Autodesk Inventor part; units mm, degrees
ref_plane "YZ Plane" through (0, 0, 0) normal (1, 0, 0) x (0, 1, 0)
ref_plane "XZ Plane" through (0, 0, 0) normal (0, 1, 0) x (-1, 0, 0)
ref_plane "XY Plane" through (0, 0, 0) normal (0, 0, 1) x (1, 0, 0)
sketch "Sketch3" plane through (0, 0, 0) normal (0, 1, 0) x (-1, 0, 0)
  line L0 (-44, 50) -> (44, 50)
  line L1 (44, 50) -> (44, -50)
  line L2 (44, -50) -> (-44, -50)
  line L3 (-44, -50) -> (-44, 50)
  line L4 (-44, 50) -> (44, -50) construction
  line L5 (44, 50) -> (-44, -50) construction
  line L6 (44, 50) -> (-44, 50)
  line L7 (-44, 50) -> (-44, 47)
  line L8 (-44, 47) -> (44, 47)
  line L9 (44, 47) -> (44, 50)
  line L10 (44, 47) -> (41, 47)
  line L11 (41, 47) -> (41, -50)
  line L12 (41, -50) -> (44, -50)
  line L13 (44, -50) -> (44, 47)
  line L14 (-44, 47) -> (-41, 47)
  line L15 (-41, 47) -> (-41, -50)
  line L16 (-41, -50) -> (-44, -50)
  line L17 (-44, -50) -> (-44, 47)
  line L18 (41, -50) -> (-41, -50)
  line L19 (-41, -50) -> (-41, -47)
  line L20 (-41, -47) -> (41, -47)
  line L21 (41, -47) -> (41, -50)
  line L22 (41, 47) -> (34, 47)
  line L23 (34, 47) -> (34, -50)
  line L24 (34, -50) -> (37, -50)
  line L25 (37, -50) -> (37, 50)
  line L26 (34, 47) -> (34, 50)
  line L27 (41, 47) -> (41, 50)
  line L28 (-41, 47) -> (-41, 50)
  point P0 (0, 0)
  point P1 (37, -47)
  point P2 (37, 47)
  point P3 (34, -47)
  point P4 (37, 50)
  dimension "d33" = 88
  dimension "d34" = 100
  dimension "d35" = 88
  dimension "d36" = 3
  dimension "d37" = 3
  dimension "d38" = 3
  dimension "d39" = 3
  dimension "d63" = 7
  dimension "d64" = 3
extrude "Extrusion2" add sketch "Sketch3" along normal blind 100 contours L8 L15 L2 L3 | L8 L25 L20 L23 | L20 L23 L2 L15 | L20 L25 L2 L23
sketch "Sketch6" plane through (44, 0, -50) normal (0, 0, -1) x (-1, 0, 0)
  circle A0 centre (62.07, 7.54) radius 1.5875
  circle A1 centre (10, 12.62) radius 1.5875
  circle A2 centre (10, 40.56) radius 1.5875
  line L0 (7.46, 10.08) -> (7.46, 42.846)
  line L1 (7.46, 42.846) -> (10, 45.386)
  line L2 (10, 45.386) -> (10, 58.34)
  line L3 (10, 7.54) -> (7.46, 10.08)
  line L4 (10, 5) -> (10, 7.54)
  line L5 (76.04, 5) -> (10, 5)
  line L6 (76.04, 58.34) -> (76.04, 5)
  line L7 (10, 58.34) -> (76.04, 58.34)
  circle A3 centre (60.8, 55.8) radius 1.5875
  line L8 (0, 0) -> (81, 0)
  line L9 (0, 100) -> (81, 100)
  line L10 (0, 0) -> (0, 100)
  line L11 (0, 0) -> (0, 100)
  line L12 (0, 0) -> (10, 0)
  line L13 (78, 0) -> (3, 0)
  line L14 (10, 0) -> (10, 5)
  line L15 (81, 0) -> (81, 100)
  point P0 (44, 0)
  point P1 (85, 0)
  dimension "d52" = 10
  dimension "d53" = 5
  dimension "d54" = 90
extrude "Extrusion4" cut sketch "Sketch6" against normal up to surface (3 mm away) contours A0 | A1 | A2 | A3
sketch "Sketch9" plane through (-37, 0, -50) normal (-1, 0, 0) x (0, 0, 1)
  line L0 (17.33, 50.02) -> (31.33, 50.02)
  line L1 (31.33, 50.02) -> (31.33, 36.02)
  line L2 (31.33, 36.02) -> (17.33, 36.02)
  line L3 (17.33, 36.02) -> (17.33, 50.02)
  line L4 (17.65, 20.175) -> (32.65, 20.175)
  line L5 (32.65, 20.175) -> (32.65, 5.175)
  line L6 (32.65, 5.175) -> (17.65, 5.175)
  line L7 (17.65, 5.175) -> (17.65, 20.175)
  point P0 (50, 0)
extrude "Extrusion6" cut sketch "Sketch9" against normal up to surface (3 mm away)
sketch "Sketch10" plane through (44, 0, 50) normal (1, 0, 0) x (0, 0, -1)
  circle A0 centre (23.979, 79.591) radius 1.0922
  circle A1 centre (62.841, 79.591) radius 1.0922
  circle A2 centre (62.841, 54.191) radius 1.0922
  line L0 (21.82, 50) -> (21.82, 81.75)
  line L1 (65, 50) -> (21.82, 50)
  line L2 (65, 81.75) -> (65, 50)
  line L3 (21.82, 81.75) -> (65, 81.75)
  circle A3 centre (23.979, 54.191) radius 1.0922
  line L4 (3, 0) -> (100, 0)
  line L5 (100, 0) -> (100, 100)
  line L6 (3, 100) -> (100, 100)
  line L7 (100, 0) -> (100, 100)
  line L8 (100, 100) -> (65, 100)
  line L9 (3, 100) -> (100, 100)
  line L10 (100, 100) -> (135, 100) construction
  line L11 (100, 0) -> (100, 100)
  line L12 (65, 100) -> (65, 0)
  line L13 (100, 0) -> (3, 0)
  line L14 (3, 0) -> (3, 100)
  point P0 (50, 0)
  point P1 (0, 0)
  point P2 (0, 100)
  dimension "d67" = 35
  dimension "d68" = 180
  dimension "d75" = 100
extrude "Extrusion7" cut sketch "Sketch10" against normal up to surface (3 mm away) contours A0 | A1 | A2 | A3
sketch "Sketch11" plane through (-37, 0, -50) normal (-1, 0, 0) x (0, 0, 1)
  circle A0 centre (75.1, 71.8) radius 1.55
  circle A1 centre (75.1, 15.4) radius 1.55
  line L0 (67.45, 5) -> (82.75, 5)
  line L1 (67.45, 82.2) -> (82.75, 82.2)
  line L2 (95, 82.2) -> (95, 5)
  line L3 (55.2, 82.2) -> (55.2, 5)
  line L4 (32.65, 5.175) -> (17.65, 5.175)
  line L5 (17.65, 5.175) -> (17.65, 20.175)
  line L6 (17.65, 20.175) -> (32.65, 20.175)
  line L7 (32.65, 20.175) -> (32.65, 5.175)
  line L8 (31.33, 50.02) -> (31.33, 36.02)
  line L9 (31.33, 36.02) -> (17.33, 36.02)
  line L10 (17.33, 36.02) -> (17.33, 50.02)
  line L11 (17.33, 50.02) -> (31.33, 50.02)
  line L12 (0, 0) -> (97, 0)
  line L13 (0, 100) -> (97, 100)
  line L14 (0, 0) -> (0, 100)
  line L15 (100, 0) -> (100, 100)
  line L16 (100, 0) -> (100, 5)
  line L17 (100, 5) -> (95, 5)
  line L18 (97, 0) -> (97, 100)
  point P0 (50, 0)
  dimension "d71" = 5
  dimension "d72" = 5
extrude "Extrusion8" cut sketch "Sketch11" against normal up to surface (3 mm away) contours A0 | A1
sketch "Sketch12" plane through (-34, 0, -47) normal (0, 0, 1) x (1, 0, 0)
  circle A0 centre (17.2, 55.8) radius 1.5875
  circle A1 centre (68, 40.56) radius 1.5875
  circle A2 centre (15.93, 7.54) radius 1.5875
  circle A3 centre (68, 12.62) radius 1.5875
  line L0 (0, 0) -> (75, 0)
  line L1 (75, 0) -> (75, 100)
  line L2 (0, 100) -> (75, 100)
  line L3 (0, 0) -> (0, 100)
  line L4 (75, 0) -> (75, 100)
  line L5 (75, 100) -> (70, 100)
  line L6 (70, 100) -> (70, 70)
  line L7 (70, 70) -> (75, 70)
  line L8 (75, 70) -> (75, 100)
  point P0 (34, 0)
  dimension "d76" = 5
  dimension "d77" = 30
extrude "Extrusion9" add sketch "Sketch12" along normal blind 2.4 contours L7 L6 L2 L1
sketch "Sketch13" plane through (-34, 0, -44.6) normal (0, 0, 1) x (1, 0, 0)
  line L0 (70, 100) -> (70, 70)
  line L1 (70, 70) -> (75, 70)
  line L2 (75, 100) -> (75, 70)
  line L3 (75, 100) -> (70, 100)
  line L4 (70, 100) -> (70, 70)
  line L5 (75, 100) -> (70, 100)
  line L6 (70, 100) -> (70, 97)
  line L7 (70, 97) -> (75, 97)
  line L8 (75, 97) -> (75, 100)
  point P0 (34, 0)
  dimension "d80" = 3
extrude "Extrusion10" add sketch "Sketch13" along normal blind 2.4 contours L3 L2 L7 L0
sketch "Sketch14" plane through (-34, 0, -47) normal (0, 0, 1) x (1, 0, 0)
  line L0 (75, 0) -> (75, 70)
  line L1 (0, 0) -> (0, 100)
  line L2 (75, 0) -> (0, 0)
  line L3 (0, 0) -> (0, 3)
  line L4 (0, 3) -> (75, 3)
  line L5 (75, 3) -> (75, 0)
  point P0 (34, 0)
  dimension "d83" = 3
extrude "Extrusion11" add sketch "Sketch14" along normal up to surface (94 mm away)
sketch "Sketch15" plane through (-37, 0, 47) normal (0, 0, 1) x (1, 0, 0)
  line L0 (0, 0) -> (81, 0)
  line L1 (81, 0) -> (81, 100)
  line L2 (78, 100) -> (81, 100)
  line L3 (78, 3) -> (78, 100)
  line L4 (3, 3) -> (78, 3)
  line L5 (3, 3) -> (3, 100)
  line L6 (0, 100) -> (3, 100)
  line L7 (0, 0) -> (0, 100)
  point P0 (37, 0)
extrude "Extrusion12" add sketch "Sketch15" along normal blind 30
sketch "Sketch16" plane through (-37, 0, -50) normal (-1, 0, 0) x (0, 0, 1)
  circle A0 centre (75.1, 15.4) radius 1.55
  circle A1 centre (75.1, 71.8) radius 1.55
  line L0 (17.65, 5.175) -> (17.65, 20.175)
  line L1 (17.65, 20.175) -> (32.65, 20.175)
  line L2 (32.65, 20.175) -> (32.65, 5.175)
  line L3 (32.65, 5.175) -> (17.65, 5.175)
  line L4 (17.33, 50.02) -> (31.33, 50.02)
  line L5 (31.33, 50.02) -> (31.33, 36.02)
  line L6 (31.33, 36.02) -> (17.33, 36.02)
  line L7 (17.33, 36.02) -> (17.33, 50.02)
  line L8 (0, 0) -> (127, 0)
  line L9 (127, 100) -> (127, 0)
  line L10 (0, 100) -> (127, 100)
  line L11 (0, 0) -> (0, 100)
  circle A2 centre (75.1, 71.8) radius 1.55
  line L12 (75.1, 71.8) -> (75.1, 91.8)
  line L13 (75.1, 91.8) -> (83.1, 91.8)
  line L14 (75.1, 91.8) -> (67.1, 91.8)
  circle A3 centre (83.1, 91.8) radius 2
  circle A4 centre (67.1, 91.8) radius 2
  line L15 (127, 3) -> (127, 100)
  line L16 (127, 51.5) -> (71.1, 51.5)
  line L17 (75.1, 11.2) -> (83.1, 11.2)
  line L18 (75.1, 11.2) -> (67.1, 11.2)
  circle A5 centre (83.1, 11.2) radius 2
  circle A6 centre (67.1, 11.2) radius 2
  line L19 (83.1, 11.2) -> (91.1, 11.2)
  line L20 (67.1, 11.2) -> (59.1, 11.2)
  line L21 (127, 3) -> (3, 3)
  circle A7 centre (59.1, 11.2) radius 2
  circle A8 centre (91.1, 11.2) radius 2
  line L22 (91.1, 11.2) -> (99.1, 11.2)
  line L23 (99.1, 11.2) -> (99.1, 21.2)
  line L24 (99.1, 21.2) -> (51.1, 21.2)
  circle A9 centre (99.1, 21.2) radius 2
  circle A10 centre (51.1, 21.2) radius 2
  point P0 (50, 0)
  dimension "d88" = 20
  dimension "d89" = 8
  dimension "d90" = 8
  dimension "d91" = 4
  dimension "d92" = 4
  dimension "d95" = 8
  dimension "d96" = 8
  dimension "d97" = 4
  dimension "d98" = 4
  dimension "d99" = 8
  dimension "d100" = 10
  dimension "d101" = 48
  dimension "d102" = 4
  dimension "d103" = 4
extrude "Extrusion13" cut sketch "Sketch16" against normal up to surface (3 mm away) contours A4 | A3 | A10 | A9 L24 L23 | L23 L24 A9
equation "\"BendRadius\" = Thickness"
equation "\"BendReliefWidth\" = Thickness"
equation "\"BendReliefDepth\" = 0.5 * Thickness"
equation "\"CornerReliefSize\" = 4 * Thickness"
equation "\"MinimumRemnant\" = 2 * Thickness"
equation "\"TransitionRadius\" = BendRadius"
equation "\"JacobiRadiusSize\" = Thickness"
equation "\"GapSize\" = Thickness"
properties part number "obudowa" material "ABS Plastic"
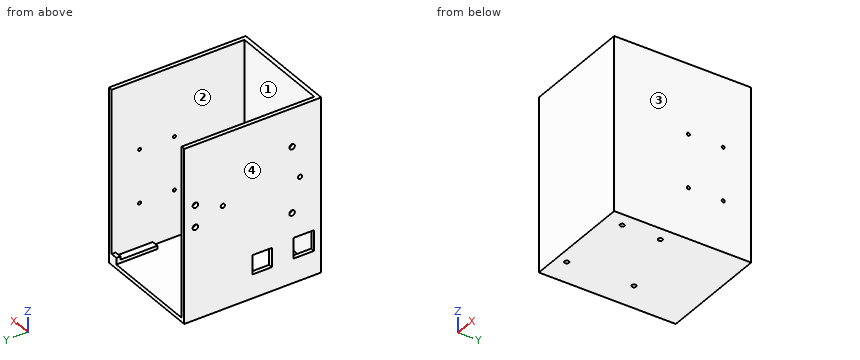
Geometry check sheet. Reference: the model listing, model coordinates, mm. Face numbers are marked on the shaded views. Coordinates: 2 decimals unless noted, no trailing zeros. Order: outer loops, then holes, each group sorted by start corner. A loop starts at its lowest first (then second) coordinate and runs counter-clockwise, first axis right, second up. Notation, with made-up numbers: (3.25, -4.75) - (33.25, -4.75) arc R20 ccw to (33.25, 13.25) - close; hole circle Ø1 at (-26, -17.5). An arc over 180 degrees is marked (long way). Answer in a Markdown table with one row per item. Add a question column.
1. Draft check along X on the marked faces 1, 2, 3 and 4. Enter one of: +X half, -X half, draft (parallel to the pull), parting line (faces both ways), or undercut.
2. Section check D-D (y = 7.54). Enter the section's corners in (x, z).
3. Section check B-B (y = 44). Enter the section's corners in (x, z).
4. Material ranges on L1, parallel to Y at x = -35, z = 25; L2, parallel to Y at x = -36.3, z = 1.1; L3, parallel to X at y = 49.5, z = -5, recorded low to high. Write a range as [from, to].
5. Section check C-C (x = 34). Enter the section's corners in (y, z), plus the area to 3 significant figures.
6. Gauge pin test, flat ends, axial feed: pin 1 Ø2.5 at (x, y) = (38.5, 99) entering from +Z; pin 2 Ø12 at (x, y) = (-17, 67.5) entering from +Z; pin 3 Ø2 at (y, z) = (54.191, 26.021) entering from +X. Record the tip position at first contact, or that the pin passes through.
7. Section check A-A (z = 1.1). Enter the section's corners in (x, y), plus the area to 3 significant figures.
Data:
| question | item | result |
|---|---|---|
| 1 | face 1 | undercut |
| 1 | face 2 | undercut |
| 1 | face 3 | +X half |
| 1 | face 4 | -X half |
| 2 | outline | (-37, -50) - (-19.66, -50) - (-19.66, -47) - (-34, -47) - (-34, -32.35) - (-37, -32.35) - close; (-37, -17.35) - (-34, -17.35) - (-34, 77) - (-37, 77) - close; (-16.48, -50) - (44, -50) - (44, 77) - (41, 77) - (41, -47) - (-16.48, -47) - close |
| 3 | outline | (-37, -50) - (44, -50) - (44, 77) - (41, 77) - (41, -47) - (-34, -47) - (-34, -32.67) - (-37, -32.67) - close; (-37, -18.67) - (-34, -18.67) - (-34, 77) - (-37, 77) - close |
| 4 | L1 | y = [0, 13.85], [16.95, 70.25], [73.35, 100] |
| 4 | L2 | y = [0, 19.2], [23.2, 100] |
| 4 | L3 | x = [-37, -34], [41, 44] |
| 5 | outline | (0, -50) - (11.03, -50) - (11.03, -47) - (3, -47) - (3, 77) - (0, 77) - close; (14.21, -50) - (38.97, -50) - (38.97, -47) - (14.21, -47) - close; (42.15, -50) - (100, -50) - (100, -47) - (42.15, -47) - close |
| 5 | area | 653 mm² |
| 6 | pin 1 | stops at z = -42.2 |
| 6 | pin 2 | stops at z = -47 |
| 6 | pin 3 | stops at x = -34 |
| 7 | outline | (-37, 0) - (44, 0) - (44, 100) - (41, 100) - (41, 3) - (-34, 3) - (-34, 19.2) - (-37, 19.2) - close; (-37, 23.2) - (-34, 23.2) - (-34, 100) - (-37, 100) - close |
| 7 | area | 813 mm² |
